The listing builds one solid part. Answer for the finished solid, in the listing's coordinates (mm). Round coordinates to 2 decimals unless told otherwise and drop trailing zeros. Order: outer loops, then holes, each group sorted by start corner. A loop starts at its lowest first (then second) coordinate and runs counter-clockwise, first axis right, second up. Notation, with made-up numbers: (44.25, 45.25) -> (83.25, 45.25) arc R31 cw to (83.25, 74.25) -> close; hole circle Ø10 at (6, 68.25). An arc over 180 degrees is marked (long way). Return JSON: item names as keys, results as strings. Group by question number.
(1) The part is cut by section A-A (x = 11.5). Determine the outline of the cut face in (y, z).
(2) This flat-tipped pin is pushed along its axis until it touches: pin 1 (1.5 mm diameter, centred on x = -0.5, z = -4.5, fed in from -Y). Where does it stop, or does it pass through?
(3) Consider line 1 (Z direction, x = -6.25, y = 1.35); line 2 (Y direction, x = -2.75, z = 9.25); line 3 (Z direction, x = 7.75, y = 0.7). Determine where each line is inside the solid, lowest interval first. Write a range as [from, to].
Autodesk Fusion 360 part; units mm, degrees
sketch "Sketch1" plane through (0, 0, 0) normal (0, 1, 0) x (1, 0, 0)
  line L0 (-15, 10) -> (15, 10)
  line L1 (15, 10) -> (15, -10)
  line L2 (15, -10) -> (-15, -10)
  line L3 (-15, -10) -> (-15, 10)
  line L4 (-15, 10) -> (15, -10) construction
  line L5 (15, 10) -> (-15, -10) construction
  dimension "d1" = 30
  dimension "d2" = 20
extrude "Extrude1" add sketch "Sketch1" along normal blind 5
fillet "Fillet1" radius 1.5 4 edges at (0, 5, 10) (0, 0, 10) (0, 5, -10) (0, 0, -10)
chamfer "Chamfer1" distance 0.5 angle 45 16 edges at (-15, 2.5, 10) (-15, 0.4393, 9.5607) (-15, 0, 0) (-15, 0.4393, -9.5607) (-15, 2.5, -10) (-15, 4.5607, -9.5607) (-15, 5, 0) (-15, 4.5607, 9.5607) (15, 2.5, -10) (15, 0.4393, -9.5607) (15, 0, 0) (15, 0.4393, 9.5607) (15, 2.5, 10) (15, 4.5607, 9.5607) (15, 5, 0) (15, 4.5607, -9.5607)
Answer below:
{
 "1": {"outline": "(0, -8.5) arc R1.5 ccw to (1.5, -10) -> (3.5, -10) arc R1.5 ccw to (5, -8.5) -> (5, 8.5) arc R1.5 ccw to (3.5, 10) -> (1.5, 10) arc R1.5 ccw to (0, 8.5) -> close"},
 "2": {"pin 1": "stops at y = 0"},
 "3": {"line 1": "z = [-9.99, 9.99]", "line 2": "y = [0.2, 4.8]", "line 3": "z = [-9.77, 9.77]"}
}
